Read the model definition and answer for the solid it produces. Units are mm, in the model's axes. A direction names the side the tool comes from. Give positions to 0.01 mm unless a question says otherwise; leave off trailing zeros. Order: outer loops, then holes, each group sorted by start corner. A loop starts at its lowest first (then second) coordinate and runs counter-clockwise, first axis right, second up.
```python
from build123d import *

# Parameters (mm, degrees)
SKETCH1_W                                       = 125
SKETCH1_H                                       = 90
BOSS_EXTRUDE1_DEPTH                             = 4
SKETCH2_R                                       = 26.25
CUT_EXTRUDE2_DEPTH                              = 78.11841544
FILLET1_R                                       = 6
FILLET2_R                                       = 2
CSK_FOR_M3_FLAT_HEAD_MACHINE_SCREW1_D           = 3.4
CSK_FOR_M3_FLAT_HEAD_MACHINE_SCREW1_CSINK_D     = 6.3
CSK_FOR_M3_FLAT_HEAD_MACHINE_SCREW1_CSINK_ANGLE = 90
CUT_EXTRUDE3_DEPTH                              = 1
M3X0_5_TAPPED_HOLE1_D                           = 2.5


with BuildPart() as part:
    # Sketch1 → Boss-Extrude1 (new body)
    with BuildSketch(Plane.XY):
        Rectangle(SKETCH1_W, SKETCH1_H)
    extrude(amount=BOSS_EXTRUDE1_DEPTH)

    # Sketch2 → Cut-Extrude2 (cut, through all)
    with BuildSketch(Plane.XY.offset(4)):
        with Locations((17.5, 0)):
            Circle(SKETCH2_R)
    extrude(amount=-CUT_EXTRUDE2_DEPTH, mode=Mode.SUBTRACT)

    # Fillet1
    fillet1_edges = [part.edges().sort_by_distance(p)[0] for p in [
        (62.5, -45, 2),
        (-62.5, -45, 2),
        (-62.5, 45, 2),
        (62.5, 45, 2),
    ]]
    fillet(fillet1_edges, radius=FILLET1_R)

    # Fillet2
    fillet2_edges = [part.edges().sort_by_distance(p)[0] for p in [
        (0, -45, 4),
        (-62.5, 0, 4),
        (62.5, 0, 4),
        (0, 45, 4),
        (-60.742640687, 43.242640687, 4),
        (60.742640687, 43.242640687, 4),
        (60.742640687, -43.242640687, 4),
        (-60.742640687, -43.242640687, 4),
    ]]
    fillet(fillet2_edges, radius=FILLET2_R)

    # CSK for M3 Flat Head Machine Screw1 (through all)
    with Locations(Plane.XY.offset(4)):
        with Locations((-56.5, 39), (56.5, 39), (56.5, -39), (-56.5, -39)):
            CounterSinkHole(CSK_FOR_M3_FLAT_HEAD_MACHINE_SCREW1_D / 2, CSK_FOR_M3_FLAT_HEAD_MACHINE_SCREW1_CSINK_D / 2, counter_sink_angle=CSK_FOR_M3_FLAT_HEAD_MACHINE_SCREW1_CSINK_ANGLE)

    # Sketch2<5> → Cut-Extrude3 (cut)
    with BuildSketch(Plane.XY.offset(4)):
        with BuildLine():
            Line((-0.275368706, 19.654166667), (14.649233321, 33.152083333))
            ThreePointArc((14.649233321, 33.152083333), (17.5, 34.25), (20.350766679, 33.152083333))
            Line((20.350766679, 33.152083333), (35.275368706, 19.654166667))
            ThreePointArc((35.275368706, 19.654166667), (44, 0), (35.275368706, -19.654166667))
            Line((35.275368706, -19.654166667), (20.350766679, -33.152083333))
            ThreePointArc((20.350766679, -33.152083333), (17.5, -34.25), (14.649233321, -33.152083333))
            Line((14.649233321, -33.152083333), (-0.275368706, -19.654166667))
            ThreePointArc((-0.275368706, -19.654166667), (-9, 0), (-0.275368706, 19.654166667))
        make_face()
    extrude(amount=-CUT_EXTRUDE3_DEPTH, mode=Mode.SUBTRACT)

    # M3x0.5 Tapped Hole1 (through all)
    with Locations(Plane.XY.offset(4)):
        with Locations((17.5, 30), (47.5, 0), (17.5, -30), (-12.5, 0)):
            Hole(M3X0_5_TAPPED_HOLE1_D / 2)


solid = part.part
```
1) Consider L1, parallel to Y at x = 17.5, z = 1.1; L2, parallel to Y at x = 56.5, z = 1.5; L3, parallel to X at y = -39, z = 1.2. Determine where each line is inside the solid, lowest interval first.
Final values:
L1: y = -45 to -31.25, -28.75 to -26.25, 26.25 to 28.75, 31.25 to 45
L2: y = -45 to -40.7, -37.3 to 37.3, 40.7 to 45
L3: x = -62.5 to -58.2, -54.8 to 54.8, 58.2 to 62.5
2) Given pin 1 (1.5 mm diameter, centred on x = -25, z = 3, fed in from +Y), flat-ended and moving along its own axis, determine where the tip first touches the part or whether it passes through.
Final values:
pin 1: stops at y = 44.98
3) The part is cut by section A-A on x = 47.5. Determine the outline of the cut face in (y, z), and give its area (3 significant figures).
Final values:
outline: (-45, 0) - (-1.25, 0) - (-1.25, 4) - (-43, 4) arc R2 ccw to (-45, 2) - close; (1.25, 0) - (45, 0) - (45, 2) arc R2 ccw to (43, 4) - (1.25, 4) - close
area: 348 mm2
4) For a pull along Y with two mould halves and no side action, classify faces 3 (the face through (4, -23, 3)), 4 (the face through (-60.789, 43.196, 1.014)), 5 (the face through (-60.789, -43.196, 1.014)), 6 (the face through (7.291, -26.498, 3.507)) as released by +Y, released by -Y, zero draft, split by the parting line, or undercut.
Final values:
face 3: undercut
face 4: released by +Y
face 5: released by -Y
face 6: undercut
5) The part is cut by section B-B on y = -17. Determine the outline of the cut face in (x, z), and give its area (3 significant figures).
Final values:
outline: (-62.5, 0) - (-2.5, 0) - (-2.5, 3) - (-2.83, 3) - (-2.83, 4) - (-60.5, 4) arc R2 ccw to (-62.5, 2) - close; (37.5, 0) - (62.5, 0) - (62.5, 2) arc R2 ccw to (60.5, 4) - (37.83, 4) - (37.83, 3) - (37.5, 3) - close
area: 338 mm2
6) The part is cut by section C-C on y = -30. Determine the outline of the cut face in (x, z).
Final values:
outline: (-62.5, 0) - (16.25, 0) - (16.25, 3) - (11.16, 3) - (11.16, 4) - (-60.5, 4) arc R2 ccw to (-62.5, 2) - close; (18.75, 0) - (62.5, 0) - (62.5, 2) arc R2 ccw to (60.5, 4) - (23.84, 4) - (23.84, 3) - (18.75, 3) - close
7) A tool of negligible diameter and unlimited length cuts with its end or side. For faces 1 (the face through (44, 0.3, 3.5)), 2 (the face through (-55.15, -40.03, 1.26)), from which of +Z, -Z, +X, -X, +Y, -Y can it reach the whole face along a straight path? Write none if from no direction.
Final values:
face 1: +Z
face 2: +Z, -Z
